Can you work these out from the model? Positions are in its coordinate system, mm. Face numbers are marked on the shaded views. A direction names the side the tool comes from. Give positions to 0.01 mm unless a question says otherwise; leave off trailing zeros. Loops run counter-clockwise (first coordinate to the right, second up) from the corner with the lowest first, then second, coordinate; pieces in that order, holes last. Notation, with made-up numbers: (-38, -22.75) - (-26, -22.75) arc R15 cw to (-26, -8.75) - close; hole circle Ø10 at (-29.75, 12.25). An arc over 180 degrees is marked (long way). Write item = value, one per line.
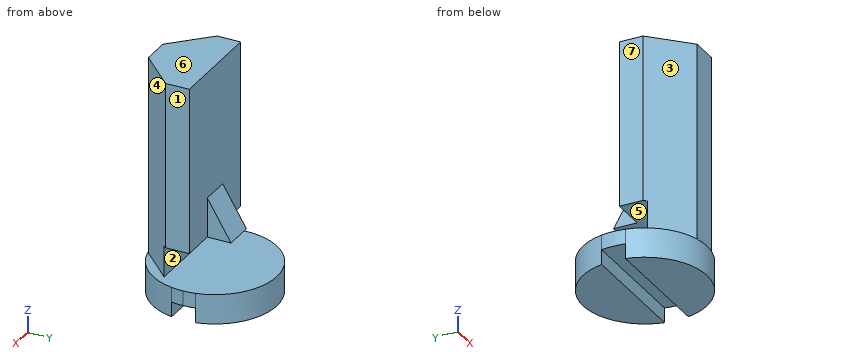
from build123d import *

# Parameters (mm, degrees)
F1_DEPTH      = 1.5
F2_DEPTH      = 0.75
F4_DEPTH      = 10
F5_T1_DEPTH   = 14.6290293783
F6_W          = 1.35
F6_H          = 1.6
F7_DEPTH      = 3.126
F7_DEPTH_BACK = 25
F9_DEPTH      = 0.75


# Not quite as in the source:
# - a fillet or chamfer that OpenCascade refuses, or shapes differently, is made with other operations: its cross-section is extruded or revolved along the edge and cut away or added


with BuildPart() as f1:
    # F0 (on Top) → F1 (new body)
    with BuildSketch(Plane.XY):
        with BuildLine():
            Line((-3.0668591425, 0.6), (3.0668591425, 0.6))
            ThreePointArc((3.0668591425, 0.6), (0, 3.125), (-3.0668591425, 0.6))
        make_face()
        with BuildLine():
            ThreePointArc((3.0668591425, -0.6), (3.1104308239, -0.3014051921), (3.125, 0))
            ThreePointArc((3.125, 0), (3.1104308239, 0.3014051921), (3.0668591425, 0.6))
            Line((3.0668591425, 0.6), (-3.0668591425, 0.6))
            ThreePointArc((-3.0668591425, 0.6), (-3.125, 0), (-3.0668591425, -0.6))
            Line((-3.0668591425, -0.6), (3.0668591425, -0.6))
        make_face()
        with BuildLine():
            ThreePointArc((-3.0668591425, -0.6), (0, -3.125), (3.0668591425, -0.6))
            Line((3.0668591425, -0.6), (-3.0668591425, -0.6))
        make_face()
    extrude(amount=F1_DEPTH)

    # F0 (on Top) → F2 (cut)
    with BuildSketch(Plane.XY):
        with BuildLine():
            ThreePointArc((3.0668591425, -0.6), (3.1104308239, -0.3014051921), (3.125, 0))
            ThreePointArc((3.125, 0), (3.1104308239, 0.3014051921), (3.0668591425, 0.6))
            Line((3.0668591425, 0.6), (-3.0668591425, 0.6))
            ThreePointArc((-3.0668591425, 0.6), (-3.125, 0), (-3.0668591425, -0.6))
            Line((-3.0668591425, -0.6), (3.0668591425, -0.6))
        make_face()
    extrude(amount=F2_DEPTH, mode=Mode.SUBTRACT)

    # F3 (on face) → F4 (join)
    with BuildSketch(Plane.XY.offset(1.5)):
        with BuildLine():
            ThreePointArc((-0.875, -3), (-1.7787811838, -2.5693505989), (-2.5, -1.875))
            Line((-2.5, -1.875), (-2.5, -3))
            Line((-2.5, -3), (-0.875, -3))
        make_face()
        with BuildLine():
            Line((2.5, 0), (-2.5, 0))
            Line((-2.5, 0), (-2.5, -1.875))
            ThreePointArc((-2.5, -1.875), (-1.7787811838, -2.5693505989), (-0.875, -3))
            Line((-0.875, -3), (0.875, -3))
            ThreePointArc((0.875, -3), (1.7787811838, -2.5693505989), (2.5, -1.875))
            Line((2.5, -1.875), (2.5, 0))
        make_face()
        with BuildLine():
            Line((2.5, -3), (2.5, -1.875))
            ThreePointArc((2.5, -1.875), (1.7787811838, -2.5693505989), (0.875, -3))
            Line((0.875, -3), (2.5, -3))
        make_face()
    extrude(amount=F4_DEPTH)

    # F5: chamfer of 1.8 on 2 edges, made by hand

    # F5_s2 → F5_t1 (cut)
    with BuildSketch(Plane.XY.offset(1.5)):
        Polygon((-2.5, -1.2), (-0.7, -3), (-2.5, -3), align=None)
        Polygon((2.5, -1.2), (0.7, -3), (2.5, -3), align=None)
    extrude(amount=F5_T1_DEPTH, mode=Mode.SUBTRACT)

    # F6 (on Right) → F7 (cut, two sides)
    with BuildSketch(Plane.YZ) as f7_sk:
        with Locations((-0.675, 2.3)):
            Rectangle(F6_W, F6_H)
    extrude(amount=-F7_DEPTH, mode=Mode.SUBTRACT)
    extrude(f7_sk.sketch, amount=F7_DEPTH_BACK, mode=Mode.SUBTRACT)

    # F8 (on Right) → F9 (join, symmetric)
    with BuildSketch(Plane.YZ):
        Polygon((0, 5.1), (0, 3.1), (1.2, 3.1), align=None)
    extrude(amount=F9_DEPTH, both=True)


solid = f1.part
Q1. For pin 1 (1.5 mm diameter, centred on y = 2.5, z = 2, fed in from -X); pin 2 (0.6 mm diameter, centred on y = 0.5, z = 3.5, fed in from -X); pin 3 (2.5 mm diameter, centred on x = 0, z = 5.5, fed in from +Y), each with a flat end and sliding along its axis, tell me the tip position at first contact or that it passes through.
Output:
pin_1 = -2.45
pin_2 = -0.75
pin_3 = 0.51
Q2. Imagine slicing it at C-C, the plane x = -1.75. Write out the boundary of the cut face in (y, z).
Output:
outline = (-2.59, 0) - (-0.6, 0) - (-0.6, 0.75) - (0.6, 0.75) - (0.6, 0) - (2.59, 0) - (2.59, 1.5) - (-1.35, 1.5) - (-1.35, 3.1) - (0, 3.1) - (0, 11.5) - (-1.95, 11.5) - (-1.95, 1.5) - (-2.59, 1.5) - close
Q3. We'd pull the mould along Z, two halves only. Please class the marked faces 5, 6 and 7: released by +Z, released by -Z, zero draft, split by the parting line, or undercut.
Output:
face_5 = undercut
face_6 = released by +Z
face_7 = zero draft
Q4. Imagine slicing it at D-D, the plane y = -1.5. Write out the boundary of the cut face in (x, z).
Output:
outline = (-2.74, 0) - (2.74, 0) - (2.74, 1.5) - (2.2, 1.5) - (2.2, 11.5) - (-2.2, 11.5) - (-2.2, 1.5) - (-2.74, 1.5) - close
Q5. Which directions (+Z, -Z, +X, -X, +Y, -Y) give clear straight access to the entire face, cutting with the end or side of a thin tool? Please do the marked faces 1, 2, 3 and 4.
Output:
face_1 = +Z, +X, +Y, -Y
face_2 = +X, -X, +Y
face_3 = +Z, -X, -Y
face_4 = +Z, +X, -Y
Q6. Imagine slicing it at A-A, the plane y = -0.25. Write out the boundary of the cut face in (x, z), then the cut area to 3 significant figures.
Output:
outline = (-3.11, 0.75) - (3.11, 0.75) - (3.11, 1.5) - (-3.11, 1.5) - close; (-2.5, 3.1) - (2.5, 3.1) - (2.5, 11.5) - (-2.5, 11.5) - close
area = 46.7 mm2
Q7. Imagine slicing it at B-B, the plane z = 4.5. Write out the boundary of the cut face in (x, y), then the cut area to 3 significant figures.
Output:
outline = (-2.5, -1.2) - (-0.7, -3) - (0.7, -3) - (2.5, -1.2) - (2.5, 0) - (0.75, 0) - (0.75, 0.36) - (-0.75, 0.36) - (-0.75, 0) - (-2.5, 0) - close
area = 12.3 mm2
Q8. I need wall thicknesses on L1, parallel to Z at x = 0.5, y = -1; L2, parallel to Z at x = 2, y = -0.5; L3, parallel to Z at x = -0.75, y = 2. Which ranges of each line are inside material? Lowest first, please.
Output:
L1 = 0 to 1.5, 3.1 to 11.5
L2 = 0.75 to 1.5, 3.1 to 11.5
L3 = 0 to 1.5
